Work out the finished part from the listing and answer in its coordinate system (mm). Round coordinates to 2 decimals unless told otherwise and drop trailing zeros. Loops run counter-clockwise (first coordinate to the right, second up) from the corner with the lowest first, then second, coordinate; pieces in that order, holes last. Notation, with made-up numbers: M 31.25,-22.5 L 50.25,-22.5 A30 cw 50.25,4.5 Z; hole C -34,18 d9. An arc over 180 degrees is marked long. One line per item, written item: value.
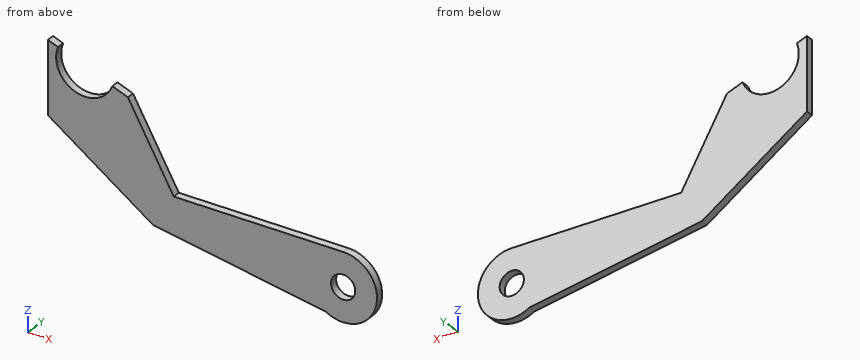
Autodesk Inventor part; units mm, degrees
ref_plane "YZ Plane" through (0, 0, 0) normal (1, 0, 0) x (0, 1, 0)
ref_plane "XZ Plane" through (0, 0, 0) normal (0, 1, 0) x (-1, 0, 0)
ref_plane "XY Plane" through (0, 0, 0) normal (0, 0, 1) x (1, 0, 0)
sketch "Szkic1" plane through (0, 0, 0) normal (0, 1, 0) x (-1, 0, 0)
  arc A0 (0, 7) -> (3.6056, -6) centre (0, 0) ccw
  line L0 (3.6056, -6) -> (39.2808, 0)
  line L1 (44.4792, 23.7708) -> (35, 7)
  line L2 (35, 7) -> (0, 7)
  circle A1 centre (0, 0) radius 2.5
  line L3 (61, 30) -> (61, 15)
  line L4 (61, 15) -> (39.2808, 0)
  arc A2 (47.6958, 24.9837) -> (58.9242, 29.2173) centre (53.31, 27.1005) ccw
  line L5 (44.4792, 23.7708) -> (47.6958, 24.9837)
  line L6 (58.9242, 29.2173) -> (61, 30)
  dimension "d0" = 14
  dimension "d1" = 5
  dimension "d5" = 12
extrude "Wyciągnięcie proste1" add sketch "Szkic1" along normal blind 1.6
properties part number "efektor szczypce1"
1) Find section C-C (y = 1.05). Give the vertices of the cut face in (x, z), then the cut area to 3 significant figures.
Check values:
outline: M -61,15 L -39.28,0 L -3.61,-6 A7 ccw long 0,7 L -35,7 L -44.48,23.77 L -47.7,24.98 A6 cw -58.92,29.22 L -61,30 Z; hole C 0,0 d5
area: 804 mm2
2) Find section D-D (z = 9). Give the vertices of the cut face in (x, y).
Check values:
outline: M -52.31,0 L -36.13,0 L -36.13,1.6 L -52.31,1.6 Z
3) Find section B-B (z = -1.5). Give the vertices of the cut face in (x, y), then the cut area to 3 significant figures.
Check values:
outline: M -30.36,0 L -2,0 L -2,1.6 L -30.36,1.6 Z; M 2,0 L 6.84,0 L 6.84,1.6 L 2,1.6 Z
area: 53.1 mm2
4) Find the intervals of material crossed by probe 1 along Z at (x, y) = (0, 0.5); probe 2 along X at (y, z) = (0.95, 2); probe 3 along X at (y, z) = (1.05, 26.5), in increasing order. Write a range as from..to.
Check values:
probe 1: -7..-2.5, 2.5..7
probe 2: -42.18..-1.5, 1.5..6.71
probe 3: -61..-59.28
5) Find section A-A (x = -1). Give the vertices of the cut face in (y, z), then the cut area to 3 significant figures.
Check values:
outline: M 0,-6.93 L 1.6,-6.93 L 1.6,-2.29 L 0,-2.29 Z; M 0,2.29 L 1.6,2.29 L 1.6,7 L 0,7 Z
area: 15.0 mm2
